The figure shows three views and two pictorial views of one solid part (mm, origin at its lowest corner). Answer the questions. A direction names the side the tool comes from. Give positions to 0.01 mm unless a question says otherwise; leave off trailing zeros. Loops run counter-clockwise (first coordinate to the right, second up) from the corner with the lowest first, then second, coordinate; pieces in that order, holes last. Notation, with made-up numbers: M 85.5,-22 L 95.5,-22 A22 cw 95.5,-14 Z; hole C 76.25,4.5 d8. An arc over 180 degrees is marked long. One line per item, written item: value. Start each with the question number.
Q1. The mould has two halves that part along X. Classify the marked faces 4, 5 and 6: +X half, -X half, draft (parallel to the pull), parting line (faces both ways), or undercut.
Q2. A cutting plane is placed at C-C, the plane z = 5.5. Determine the outline of the cut face in (x, y).
Q3. For the marked faces 1, 2 and 3, determine the directions among +Z, -Z, +X, -X, +Y, -Y from which every point of the face is accessible in a straight line to the end or side of a thin tool.
Q4. A cutting plane is placed at B-B, the plane x = 52. Determine the outline of the cut face in (y, z).
Q5. A cutting plane is placed at D-D, the plane y = 19. Determine the outline of the cut face in (x, z).
Q6. Flat-ended cylindrical pins translate along their axes: pin 1 (2 mm diameter, centred on y = 6, z = 9, fed in from -X) (3 decimals); pin 2 (7.5 mm diameter, centred on x = 44.5, y = 26, fed in from -Z); pin 3 (12 mm diameter, centred on y = 43.5, z = 44.5, fed in from +X); pin 4 (4 mm diameter, centred on x = 40.5, z = 9, fed in from -Y). Find the tip coordinate at first contact, or state that the pin passes through.
Q7. Consider L1, parallel to X at y = 16, z = 9; L2, parallel to Y at x = 45, z = 46.5; L3, parallel to Z at x = 53.5, y = 44. Determine where each line is inside the solid, lowest interval first.
Q8. A cutting plane is placed at A-A, the plane y = 10.5. Determine the outline of the cut face in (x, z).
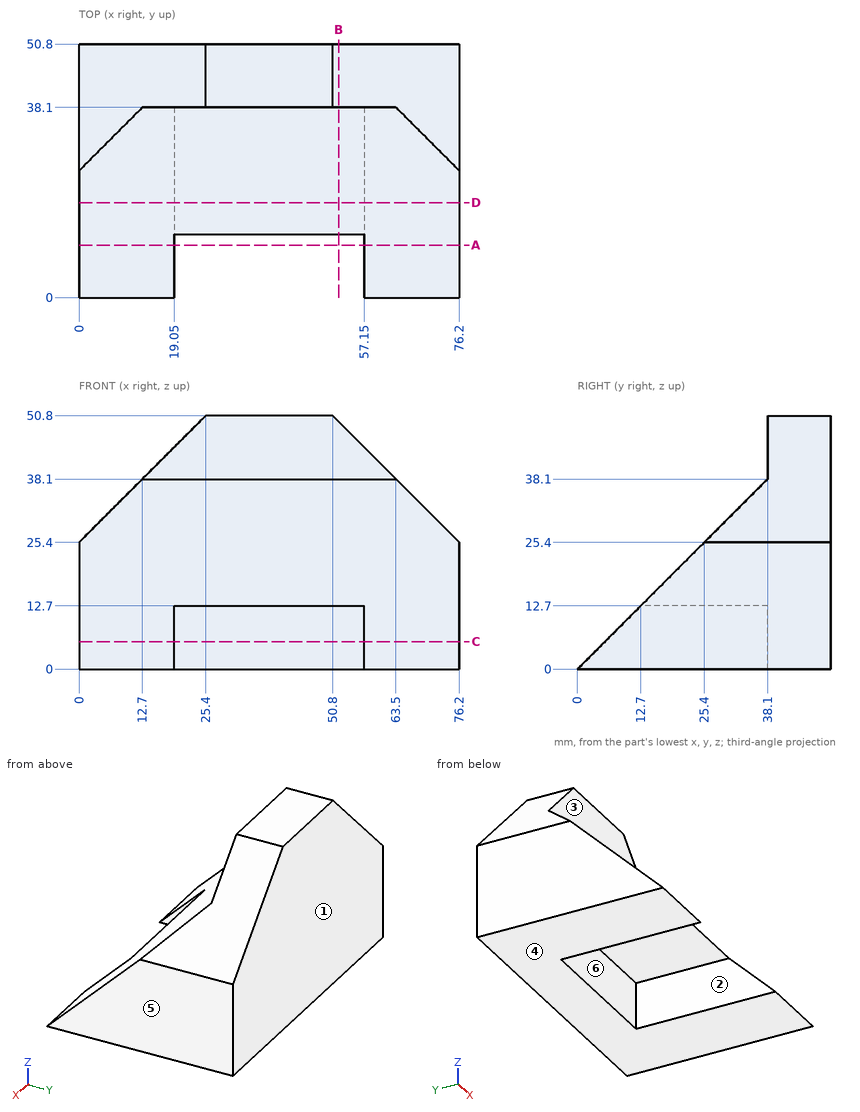
Answer block:
1. face 4: draft
1. face 5: +X half
1. face 6: undercut
2. outline: M 0,5.5 L 19.05,5.5 L 19.05,38.1 L 57.15,38.1 L 57.15,5.5 L 76.2,5.5 L 76.2,50.8 L 0,50.8 Z
3. face 1: +Z, -Z, +X, -X, +Y
3. face 2: -Z, -Y
3. face 3: +Z, +X, -X, -Y
4. outline: M 12.7,12.7 L 38.1,12.7 L 38.1,0 L 50.8,0 L 50.8,49.6 L 38.1,49.6 L 38.1,38.1 Z
5. outline: M 0,0 L 19.05,0 L 19.05,12.7 L 57.15,12.7 L 57.15,0 L 76.2,0 L 76.2,19 L 0,19 Z
6. pin 1: through
6. pin 2: z = 12.7
6. pin 3: x = 63.1
6. pin 4: y = 38.1
7. L1: 0 to 19.05, 57.15 to 76.2
7. L2: 38.1 to 50.8
7. L3: 0 to 48.1
8. outline: M 0,0 L 19.05,0 L 19.05,10.5 L 0,10.5 Z; M 57.15,0 L 76.2,0 L 76.2,10.5 L 57.15,10.5 Z
